Design review of the part built by this model. Coordinates are the model's own, in mm. Give positions to 0.01 mm unless a question says otherwise; leave off trailing zeros. Order: outer loops, then holes, each group sorted by start corner. A loop starts at its lowest first (then second) coordinate and runs counter-clockwise, first axis right, second up. Notation, with made-up numbers: (48.25, 14.5) -> (61.25, 14.5) arc R25 cw to (61.25, 44.5) -> close; hole circle Ø6 at (84.25, 61.5). An arc over 180 degrees is marked (long way). Use a Markdown table: item, result. Add a question column.
```python
from build123d import *

# Parameters (mm, degrees)
F0_R     = 34.5
F0_R_2   = 2
F1_DEPTH = 8


with BuildPart() as f1:
    # F0 (on Top) → F1 (new body)
    with BuildSketch(Plane.XY):
        Circle(F0_R)
        with BuildLine():
            ThreePointArc((0, 22), (15.5563491861, 15.5563491861), (22, 0))
            ThreePointArc((22, 0), (15.5563491861, -15.5563491861), (0, -22))
            ThreePointArc((0, -22), (-22, 0), (0, 22))
        make_face(mode=Mode.SUBTRACT)
        with BuildLine():
            ThreePointArc((0, -22), (15.5563491861, -15.5563491861), (22, 0))
            ThreePointArc((22, 0), (15.5563491861, 15.5563491861), (0, 22))
            ThreePointArc((0, 22), (-22, 0), (0, -22))
        make_face()
        with BuildLine():
            ThreePointArc((4.5, -17.5), (3.1819805153, -20.6819805153), (0, -22))
            ThreePointArc((0, -22), (-3.1819805153, -14.3180194847), (4.5, -17.5))
        make_face(mode=Mode.SUBTRACT)
        Circle(F0_R_2, mode=Mode.SUBTRACT)
        with BuildLine():
            ThreePointArc((4.5, 17.5), (-3.1819805153, 14.3180194847), (0, 22))
            ThreePointArc((0, 22), (3.1819805153, 20.6819805153), (4.5, 17.5))
        make_face(mode=Mode.SUBTRACT)
    extrude(amount=F1_DEPTH)


solid = f1.part
```
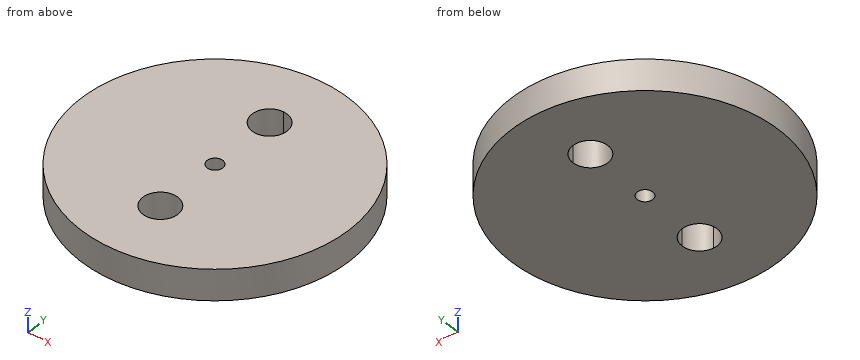
1) For L1, parallel to Y at x = 0, z = 3.5; L2, parallel to X at y = -1, z = 1; L3, parallel to X at y = 19.5, z = 7.5, list the stretches that pass through material, from the lowest coordinate up. Write a range as [from, to].
2) Add section B-B (z = 4.5). Give the boundary of the cut face in (x, y), then the cut area to 3 significant figures.
3) Add section A-A (y = 0). Give the boundary of the cut face in (x, z).
4) Insertion check: pin 1 (3 mm diameter, centred on x = 0, y = 0, fed in from +Z); pin 2 (3 mm diameter, centred on y = 25.5, z = 4.5, fed in from +X); pin 3 (1 mm diameter, centred on x = -5, z = 4.5, fed in from -Y); pin 4 (3 mm diameter, centred on y = -3, z = 6.5, fed in from -X). Each pin has a flat end and moves straight along its axis. Give the tip position at first contact, or say it passes through.
5) Add section D-D (y = 23.5). Give the boundary of the cut face in (x, z), then the cut area to 3 significant figures.
6) Add section C-C (x = 21). Give the boundary of the cut face in (y, z).
Worked answers:
| question | item | result |
|---|---|---|
| 1 | L1 | [-34.5, -22], [-13, -2], [2, 13], [22, 34.5] |
| 1 | L2 | [-34.49, -1.73], [1.73, 34.49] |
| 1 | L3 | [-28.46, -4.03], [4.03, 28.46] |
| 2 | outline | circle Ø69 at (0, 0); hole circle Ø9 at (0, -17.5); hole circle Ø9 at (0, 17.5); hole circle Ø4 at (0, 0) |
| 2 | area | 3,600 mm^2 |
| 3 | outline | (-34.5, 0) -> (-2, 0) -> (-2, 8) -> (-34.5, 8) -> close; (2, 0) -> (34.5, 0) -> (34.5, 8) -> (2, 8) -> close |
| 4 | pin 1 | through |
| 4 | pin 2 | x = 24.78 |
| 4 | pin 3 | y = -34.21 |
| 4 | pin 4 | x = -34.47 |
| 5 | outline | (-25.26, 0) -> (25.26, 0) -> (25.26, 8) -> (-25.26, 8) -> close |
| 5 | area | 404 mm^2 |
| 6 | outline | (-27.37, 0) -> (27.37, 0) -> (27.37, 8) -> (-27.37, 8) -> close |
